```python
from build123d import *

# Parameters (mm, degrees)
F0_R     = 38.1
F1_DEPTH = 15.24
F3_SCALE = 1.5


with BuildPart() as f1:
    # F0 (on Top) → F1 (new body)
    with BuildSketch(Plane.XY):
        with Locations((-42.0107929352, 37.7116280534)):
            Circle(F0_R)
        with BuildLine():
            ThreePointArc((-23.7545429352, 69.332380609), (-10.3900403795, 55.9678780534), (-5.4982929352, 37.7116280534))
            ThreePointArc((-5.4982929352, 37.7116280534), (-10.3900403795, 19.4553780534), (-23.7545429352, 6.0908754977))
            ThreePointArc((-23.7545429352, 6.0908754977), (-42.0107929352, 1.1991280534), (-60.2670429352, 6.0908754977))
            ThreePointArc((-60.2670429352, 6.0908754977), (-73.6315454908, 19.4553780534), (-78.5232929352, 37.7116280534))
            ThreePointArc((-78.5232929352, 37.7116280534), (-73.6315454908, 55.9678780534), (-60.2670429352, 69.332380609))
            ThreePointArc((-60.2670429352, 69.332380609), (-42.0107929352, 74.2241280534), (-23.7545429352, 69.332380609))
        make_face(mode=Mode.SUBTRACT)
    extrude(amount=F1_DEPTH)


with BuildPart() as f1_1:
    # F3: moved
    add(f1.part.scale(F3_SCALE).moved(Location((21.0048016161, -18.8555214554, 0))))


solid = f1_1.part
```
Read the model definition and answer for the solid it produces. Units are mm, in the model's axes. Coordinates: 2 decimals unless noted, no trailing zeros. Loops run counter-clockwise (first coordinate to the right, second up) from the corner with the lowest first, then second, coordinate; pieces in that order, holes last. Notation, with made-up numbers: (6.5, 39.25) -> (57.5, 39.25) arc R19 cw to (57.5, 74.25) -> close; hole circle Ø10 at (-13.5, 58.5). An arc over 180 degrees is marked (long way). Return JSON: item names as keys, results as strings.
Item 1: Find section B-B (y = 86.5). Determine the outline of the cut face in (x, z).
Answers:
{"outline": "(-71.77, 0) -> (-66.9, 0) -> (-66.9, 22.86) -> (-71.77, 22.86) -> close; (-17.12, 0) -> (-12.25, 0) -> (-12.25, 22.86) -> (-17.12, 22.86) -> close"}
Item 2: Flat-ended cylindrical pins translate along their axes: P1, Ø3, axis at y = 81, z = 14.5, coming from the -X side; P2, Ø10, axis at x = -9, y = 76, coming from the -Z side; P3, Ø10, axis at y = 68.5, z = 5.5, coming from the -X side; P4, Ø8, axis at x = -54, z = 4, coming from the +Y side. Find the tip coordinate at first contact, or state that the pin passes through.
Answers:
{"P1": "stops at x = -81", "P2": "stops at z = 0", "P3": "stops at x = -93.01", "P4": "stops at y = 94.3"}
Item 3: Find section A-A (x = -6). Determine the outline of the cut face in (y, z).
Answers:
{"outline": "(-6.66, 0) -> (-3.55, 0) -> (-3.55, 22.86) -> (-6.66, 22.86) -> close; (78.98, 0) -> (82.09, 0) -> (82.09, 22.86) -> (78.98, 22.86) -> close"}
Item 4: Find the intervals of material crossed by probe 1 along X at (y, z) = (38.5, 1.5); probe 2 along X at (y, z) = (0, 16); probe 3 along Y at (x, z) = (-58, 11), in increasing order.
Answers:
{"probe 1": "x = -99.16 to -96.77, 12.75 to 15.13", "probe 2": "x = -84.95 to -81.73, -2.29 to 0.93", "probe 3": "y = -17.16 to -14.67, 90.09 to 92.58"}
Item 5: Find section C-C (z = 16). Determine the outline of the cut face in (x, y).
Answers:
{"outline": "circle Ø114.3 at (-42.01, 37.71); hole circle Ø109.54 at (-42.01, 37.71)"}
